Work out the finished part from the listing and answer in its coordinate system (mm). Face numbers are marked on the shaded views. A direction names the side the tool comes from. Round coordinates to 2 decimals unless told otherwise and drop trailing zeros. Write each loop counter-clockwise with the first axis right and the second up, starting at its lowest first coordinate (ties: lowest second). Pieces come first, ordered by that corner, then holes. Notation, with made-up numbers: M -9.5,63 L 30.5,63 A17 ccw 30.5,90 Z; hole C -19.5,45 d10. An arc over 180 degrees is marked long. Answer in a Markdown table with one row per item.
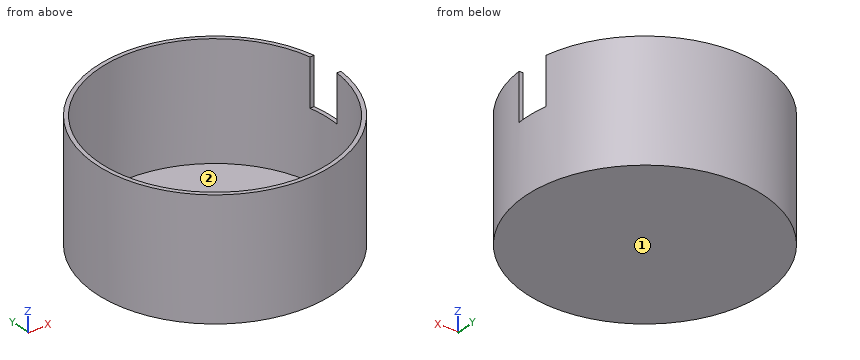
```python
from build123d import *

# Parameters (mm, degrees)
SKETCH1_R           = 150
BOSS_EXTRUDE1_DEPTH = 150
SHELL2_T            = -5
SKETCH4_W           = 60
SKETCH4_H           = 40
CUT_EXTRUDE1_DEPTH  = 150


with BuildPart() as part:
    # Sketch1 → Boss-Extrude1 (new body)
    with BuildSketch(Plane.XY):
        Circle(SKETCH1_R)
    extrude(amount=BOSS_EXTRUDE1_DEPTH)

    # Shell2
    shell2_openings = [part.faces().sort_by_distance(p)[0] for p in [
        (0, 0, 150),
    ]]
    offset(amount=SHELL2_T, openings=shell2_openings, kind=Kind.INTERSECTION)

    # Sketch4 → Cut-Extrude1 (cut)
    with BuildSketch(Plane(origin=(0, 0, 0), x_dir=(0, 0, -1), z_dir=(1, 0, 0))):
        with Locations((-120.445229028, 9.94063613)):
            Rectangle(SKETCH4_W, SKETCH4_H)
    extrude(amount=CUT_EXTRUDE1_DEPTH, mode=Mode.SUBTRACT)


solid = part.part
```
1. Given pin 1 (8 mm diameter, centred on x = 6.5, y = 99, fed in from +Z); pin 2 (10 mm diameter, centred on y = 47.5, z = 97, fed in from -X); pin 3 (10 mm diameter, centred on y = 83, z = 116.5, fed in from -X), each flat-ended and moving along its own axis, determine where each tip first touches the part or whether it passes through.
Calculated:
| item | result |
|---|---|
| pin 1 | stops at z = 5 |
| pin 2 | stops at x = -143.85 |
| pin 3 | stops at x = -128.12 |
2. The part is cut by section C-C (y = 0). Determine the outline of the cut face in (x, z).
Calculated:
| item | result |
|---|---|
| outline | M -150,0 L 150,0 L 150,90.45 L 145,90.45 L 145,5 L -145,5 L -145,150 L -150,150 Z |
3. The part is cut by section D-D (z = 105.5). Determine the outline of the cut face in (x, y), plus the area to 3 significant figures.
Calculated:
| item | result |
|---|---|
| outline | M 141.88,29.94 L 146.98,29.94 A150 ccw long 149.66,-10.06 L 144.65,-10.06 A145 cw long Z |
| area | 4,430 mm² |
4. A tool of negligible diameter and unlimited length cuts with its end or side. For the marked faces 1 and 2, from which of +Z, -Z, +X, -X, +Y, -Y can it reach the whole face along a straight path? Write none if from no direction.
Calculated:
| item | result |
|---|---|
| face 1 | -Z, +X, -X, +Y, -Y |
| face 2 | +Z |
5. The part is cut by section B-B (z = 50.5). Determine the outline of the cut face in (x, y), plus the area to 3 significant figures.
Calculated:
| item | result |
|---|---|
| outline | C 0,0 d300; hole C 0,0 d290 |
| area | 4,630 mm² |
6. Consider line 1 along Y through (x, z) = (0, 69); line 2 along Z through (x, y) = (78, 43). Determine where each line is inside the solid, lowest interval first. Write a range as from..to.
Calculated:
| item | result |
|---|---|
| line 1 | y = -150..-145, 145..150 |
| line 2 | z = 0..5 |
7. The part is cut by section A-A (x = 0). Determine the outline of the cut face in (y, z), plus the area to 3 significant figures.
Calculated:
| item | result |
|---|---|
| outline | M -150,0 L 150,0 L 150,150 L 145,150 L 145,5 L -145,5 L -145,150 L -150,150 Z |
| area | 2,950 mm² |
